For this review, take the finished solid that the model builds, in its own axes (mm). Face numbers are marked on the shaded views. A direction names the side the tool comes from. Round coordinates to 2 decimals unless told otherwise and drop trailing zeros. Order: outer loops, then holes, each group sorted by start corner. A loop starts at its lowest first (then second) coordinate and runs counter-clockwise, first axis right, second up. Notation, with made-up numbers: (73, 3) - (78, 3) arc R9 cw to (78, 7) - close; hole circle Ø5 at (-17, 81.5). An arc over 180 degrees is marked (long way). One line per item, written item: value.
Autodesk Inventor part; units mm, degrees
ref_plane "YZ Plane" through (0, 0, 0) normal (1, 0, 0) x (0, 1, 0)
ref_plane "XZ Plane" through (0, 0, 0) normal (0, 1, 0) x (-1, 0, 0)
ref_plane "XY Plane" through (0, 0, 0) normal (0, 0, 1) x (1, 0, 0)
sketch "Sketch1" plane through (0, 0, 0) normal (0, 0, 1) x (1, 0, 0)
  line L0 (0, 0) -> (19, 0)
  line L1 (19, 0) -> (19, 9)
  line L2 (19, 9) -> (0, 9)
  line L3 (0, 9) -> (0, 0)
  point P0 (9.5, 9)
  dimension "d0" = 19
  dimension "d1" = 9
extrude "Extrusion1" add sketch "Sketch1" along normal blind 3
sketch "Sketch2" plane through (0, 0, 3) normal (0, 0, 1) x (1, 0, 0)
  line L0 (19, 9) -> (0, 9)
  circle A0 centre (9.5, 7) radius 1
  point P0 (0, 0)
  point P1 (9.5, 9)
  dimension "d4" = 2
  dimension "d5" = 2
extrude "Extrusion2" add sketch "Sketch2" along normal blind 3.5
sketch "Sketch6" plane through (9.5, 7, 6.5) normal (0, 0, 1) x (1, 0, 0)
  circle A0 centre (0, 0) radius 1
  line L0 (2, -1) -> (-2, -1)
  line L1 (-2, -1) -> (-2, 1)
  line L2 (-2, 1) -> (2, 1)
  line L3 (2, 1) -> (2, -1)
  line L4 (2, -1) -> (-2, 1) construction
  line L5 (-2, -1) -> (2, 1) construction
  point P0 (-9.5, -7)
  dimension "d13" = 4
extrude "Extrusion5" add sketch "Sketch6" along normal blind 32
sketch "Sketch7" plane through (9.5, 7, 38.5) normal (0, 0, 1) x (1, 0, 0)
  circle A0 centre (0, 0) radius 1
  line L0 (-9.5, -7) -> (9.5, -7)
  line L1 (9.5, -7) -> (9.5, 2)
  line L2 (9.5, 2) -> (-9.5, 2)
  line L3 (-9.5, 2) -> (-9.5, -7)
  arc A1 (0, -1) -> (0, 1) centre (0, 0) ccw
  arc A2 (0, 1) -> (0, -1) centre (0, 0) ccw
extrude "Extrusion6" add sketch "Sketch7" along normal blind 4 contours A0 | L3 L2 L1 L0
sketch "Sketch8" plane through (9.5, 7, 42.5) normal (0, 0, 1) x (1, 0, 0)
  line L0 (-9.5, -7) -> (9.5, -7)
  line L1 (9.5, -7) -> (9.5, 2)
  line L2 (9.5, 2) -> (-9.5, 2)
  line L3 (-9.5, 2) -> (-9.5, -7)
  circle A0 centre (0, -2.5) radius 1.65
  dimension "d18" = 3.3
extrude "Extrusion7" cut sketch "Sketch8" against normal blind 4 contours A0
sketch "Sketch10" plane through (0, 0, 0) normal (-1, 0, 0) x (0, 0, 1)
  line L0 (0, 0) -> (3, 0)
  line L1 (3, 9) -> (3, 0)
  line L2 (3, 0) -> (2, 0)
  line L3 (2, 0) -> (2, 6)
  line L4 (2, 6) -> (3, 6)
  line L5 (3, 6) -> (3, 0)
  line L6 (3, 0) -> (2, 1)
  line L7 (3, 0) -> (4.4142, 0) construction
  line L8 (2, 1) -> (3, 2)
  line L9 (3, 0) -> (3, 9)
  line L10 (3, 2) -> (2, 3)
  line L11 (2, 3) -> (3, 4)
  line L12 (2, 5) -> (3, 4)
  line L13 (2, 5) -> (3, 6)
  dimension "d23" = 1
  dimension "d24" = 6
  dimension "d25" = 135
  dimension "d26" = 90
extrude "Extrusion8" cut sketch "Sketch10" against normal up to next contours L6 L8 L1 | L10 L11 L1 | L12 L13 L1
sketch "Sketch11" plane through (0, 0, 0) normal (0, -1, 0) x (1, 0, 0)
  line L0 (0, 3) -> (9.5, 3)
  line L1 (0, 3) -> (19, 3)
  line L2 (19, 3) -> (19, 2)
  line L3 (19, 2) -> (8.5, 2)
  line L4 (0, 2) -> (0, 3)
  line L5 (0, 3) -> (0, 2)
  line L6 (0, 3) -> (1.4142, 3) construction
  line L7 (19, 3) -> (0, 3)
  line L8 (9.5, 3) -> (8.5, 2)
  line L9 (9.5, 3) -> (10.9142, 3) construction
  line L10 (10.5, 2) -> (8.5, 2)
  line L11 (9.5, 3) -> (10.5, 2)
  line L12 (10.5, 2) -> (8.5, 2)
  line L13 (8.5, 2) -> (0, 2)
  line L14 (7.5, 3) -> (8.5, 2)
  line L15 (8.5, 2) -> (6.5, 2)
  line L16 (7.5, 3) -> (6.5, 2)
  line L17 (5.5, 3) -> (6.5, 2)
  line L18 (6.5, 2) -> (4.5, 2)
  line L19 (5.5, 3) -> (4.5, 2)
  line L20 (3.5, 3) -> (4.5, 2)
  line L21 (4.5, 2) -> (2.5, 2)
  line L22 (3.5, 3) -> (2.5, 2)
  line L23 (12.5, 2) -> (10.5, 2)
  line L24 (11.5, 3) -> (12.5, 2)
  line L25 (11.5, 3) -> (10.5, 2)
  line L26 (14.5, 2) -> (12.5, 2)
  line L27 (13.5, 3) -> (14.5, 2)
  line L28 (13.5, 3) -> (12.5, 2)
  line L29 (16.5, 2) -> (14.5, 2)
  line L30 (15.5, 3) -> (16.5, 2)
  line L31 (15.5, 3) -> (14.5, 2)
  point P0 (0, 0)
  dimension "d30" = 135
  dimension "d33" = 2
  dimension "d40" = 2
extrude "Extrusion9" cut sketch "Sketch11" against normal blind 6 contours L0 L22 L13 L4 | L0 L19 L20 | L0 L16 L17 | L0 L8 L14 | L1 L25 L11 | L1 L28 L24 | L1 L31 L27 | L1 L2 L3 L30
fillet "Fillet2" radius 1 4 edges at (19, 0, 1) (19, 9, 1.5) (0, 0, 1) (0, 9, 1.5)
fillet "Fillet3" radius 2 4 edges at (19, 0, 40.5) (19, 9, 40.5) (0, 0, 40.5) (0, 9, 40.5)
chamfer "Chamfer1" distance 1 distance2 3 1 edges at (7.5, 7, 6.5) measured on face at (7.8358, 6.9598, 6.5)
chamfer "Chamfer2" distance 1 distance2 3 1 edges at (11.5, 7, 6.5) measured on face at (11.1667, 7, 6.5)
properties part number "gravity-clamp-base9x19mm-part1"
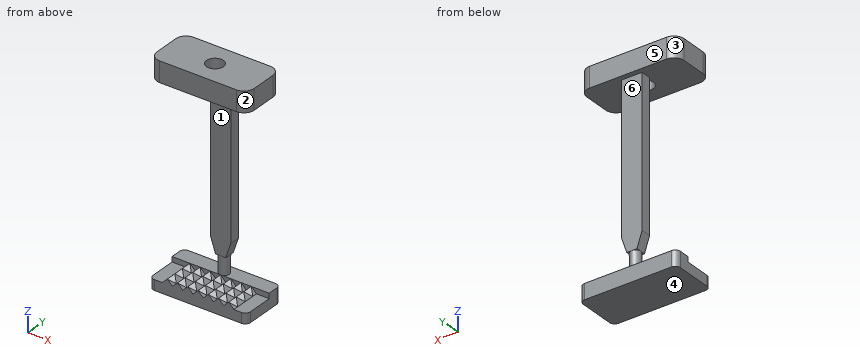
Item 1: For P1, Ø0.8, axis at x = 9, z = 2.5, coming from the -Y side; P2, Ø1.2, axis at x = 10.5, z = 21, coming from the -Y side; P3, Ø1, axis at y = 6.5, z = 19.5, coming from the +X side; P4, Ø2, axis at y = 7.5, z = 18.5, coming from the -X side, all flat-tipped, find the tip position at first contact; note any pin that passes through.
Returned:
P1: y = 0
P2: y = 6
P3: x = 11.5
P4: x = 7.5
Item 2: Take a section at B-B (z = 20). Write out the cut boundary in (x, y), plus the area to 3 significant figures.
Returned:
outline: (7.5, 6) - (11.5, 6) - (11.5, 8) - (7.5, 8) - close
area: 8.00 mm^2
Item 3: Wall thickness on line 1 (Y direction, x = 9.5, z = 39.6); line 2 (X direction, y = 4.5, z = 39.6); line 3 (Z direction, x = 14, y = 7.75): over which ranges is each line inside the solid? List them lowest first.
Returned:
line 1: 0 to 2.85, 6.15 to 9
line 2: 0 to 7.85, 11.15 to 19
line 3: 0 to 3, 38.5 to 42.5
Item 4: Take a section at A-A (y = 4.5). Count the separate pieces of the cut face and the enclosed holes in it, plus the area to 3 significant figures.
Returned:
separate pieces: 3
enclosed holes: 0
area: 106 mm^2
Item 5: The part is to be moulded in two halves that separate along Z. For the marked faces 4, 5 and 6, say which applies: +Z half, -Z half, draft (parallel to the pull), parting line (faces both ways), or undercut.
Returned:
face 4: -Z half
face 5: draft
face 6: undercut
Item 6: Machinability: for the marked faces 1, 2 and 3, which of the approach directions +Z, -Z, +X, -X, +Y, -Y give a long, thin tool a straight path to every point of the face, cutting with its end or side? Answer none if there is none.
Returned:
face 1: +X, -X, -Y
face 2: +Z, +X, -Y
face 3: +Z, -X, +Y
